from build123d import *

# Parameters (mm, degrees)
F1_DEPTH = 250
F3_DEPTH = 25
F4_R     = 13
F5_DEPTH = 25


with BuildPart() as f1:
    # F0 (on Front) → F1 (new body)
    with BuildSketch(Plane.XZ):
        Polygon((-28.448276, 1.130267), (-28.448276, 0), (-28.448276, -18.869733), (21.551724, -18.869733), (21.551724, 1.130267), align=None)
    extrude(amount=F1_DEPTH)

    # F2 (on face) → F3 (cut)
    with BuildSketch(Plane.XY.offset(1.130267)):
        with BuildLine():
            Line((21.551724, 0), (-3.448276, 0))
            ThreePointArc((-3.448276, 0), (14.229393, -7.32233), (21.551724, -25))
            Line((21.551724, -25), (21.551724, 0))
        make_face()
        with BuildLine():
            Line((-28.448276, 0), (-28.448276, -25))
            ThreePointArc((-28.448276, -25), (-21.125946, -7.32233), (-3.448276, 0))
            Line((-3.448276, 0), (-28.448276, 0))
        make_face()
        with BuildLine():
            ThreePointArc((21.551724, -225), (14.229393, -242.67767), (-3.448277, -250))
            Line((-3.448277, -250), (21.551724, -250))
            Line((21.551724, -250), (21.551724, -225))
        make_face()
        with BuildLine():
            ThreePointArc((-3.448277, -250), (-21.125946, -242.677669), (-28.448276, -225))
            Line((-28.448276, -225), (-28.448276, -250))
            Line((-28.448276, -250), (-3.448277, -250))
        make_face()
    extrude(amount=-F3_DEPTH, mode=Mode.SUBTRACT)

    # F4 (on face) → F5 (cut)
    with BuildSketch(Plane.XY.offset(1.130267)):
        with Locations((-3.448276, -20)):
            Circle(F4_R)
        with Locations((-3.448276, -230)):
            Circle(F4_R)
    extrude(amount=-F5_DEPTH, mode=Mode.SUBTRACT)


solid = f1.part
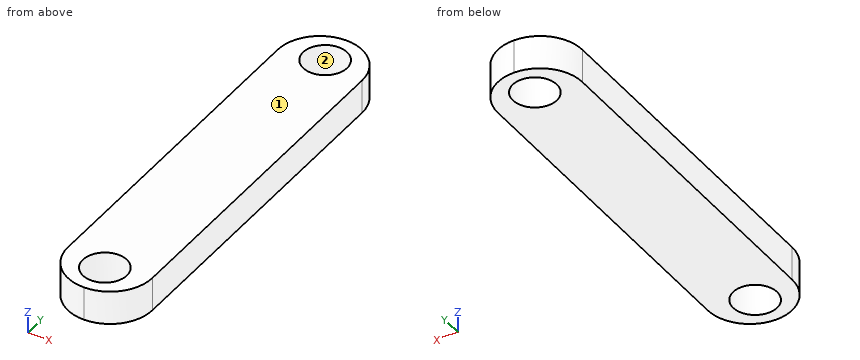
Part model, mm, in its own coordinate system. Face numbers are marked on the shaded views. Give positions to 0.01 mm unless a question says otherwise; leave off trailing zeros. Order: outer loops, then holes, each group sorted by start corner. A loop starts at its lowest first (then second) coordinate and runs counter-clockwise, first axis right, second up. Notation, with made-up numbers: (59.25, 11.5) - (111.25, 11.5) arc R23 ccw to (111.25, 26.5) - close; hole circle Ø5 at (72.5, 77.5). An arc over 180 degrees is marked (long way). Use a Markdown table: item, result.
1) Saw through at D-D on x = -23. List the corners of the cut face in (y, z), plus the area to 3 significant figures.
Checked values:
| item | result |
|---|---|
| outline | (-240.58, -18.87) - (-9.42, -18.87) - (-9.42, 1.13) - (-240.58, 1.13) - close |
| area | 4,620 mm² |
2) Saw through at A-A on y = -20. List the corners of the cut face in (x, z).
Checked values:
| item | result |
|---|---|
| outline | (-27.94, -18.87) - (-16.45, -18.87) - (-16.45, 1.13) - (-27.94, 1.13) - close; (9.55, -18.87) - (21.05, -18.87) - (21.05, 1.13) - (9.55, 1.13) - close |
3) Probe L1, parallel to Y at x = -2.5, z = -6.5; L2, parallel to Y at x = -7.5, z = -5.25; L3, parallel to Y at x = 17.5, z = -10. List the from-to ranges inside material, lowest first. Write a range as from..to.
Checked values:
| item | result |
|---|---|
| L1 | -249.98..-242.97, -217.03..-32.97, -7.03..-0.02 |
| L2 | -249.67..-242.35, -217.65..-32.35, -7.65..-0.33 |
| L3 | -238.64..-11.36 |
4) Two-plate mould, pull along Y, no slides. Class the marked faces 1 and 2: +Y half, -Y half, draft (parallel to the pull), parting line (faces both ways), or undercut.
Checked values:
| item | result |
|---|---|
| face 1 | draft |
| face 2 | undercut |
5) Saw through at C-C on z = -2.5. List the corners of the cut face in (x, y), plus the area to 3 significant figures.
Checked values:
| item | result |
|---|---|
| outline | (-28.45, -225) arc R25 ccw to (21.55, -225) - (21.55, -25) arc R25 ccw to (-3.45, 0) arc R25 ccw to (-28.45, -25) - close; hole circle Ø26 at (-3.45, -230); hole circle Ø26 at (-3.45, -20) |
| area | 10,900 mm² |
6) Saw through at B-B on x = 0. List the corners of the cut face in (y, z), plus the area to 3 significant figures.
Checked values:
| item | result |
|---|---|
| outline | (-249.76, -18.87) - (-242.53, -18.87) - (-242.53, 1.13) - (-249.76, 1.13) - close; (-217.47, -18.87) - (-32.53, -18.87) - (-32.53, 1.13) - (-217.47, 1.13) - close; (-7.47, -18.87) - (-0.24, -18.87) - (-0.24, 1.13) - (-7.47, 1.13) - close |
| area | 3,990 mm² |
7) Flat gauge pins, fed straight in: P1, Ø2, axis at x = 2, z = -12, coming from the +Y side; P2, Ø3, axis at x = 4, z = -3, coming from the -Y side. Where does each tip first touch, or does it go through?
Checked values:
| item | result |
|---|---|
| P1 | y = -0.4 |
| P2 | y = -249.28 |
